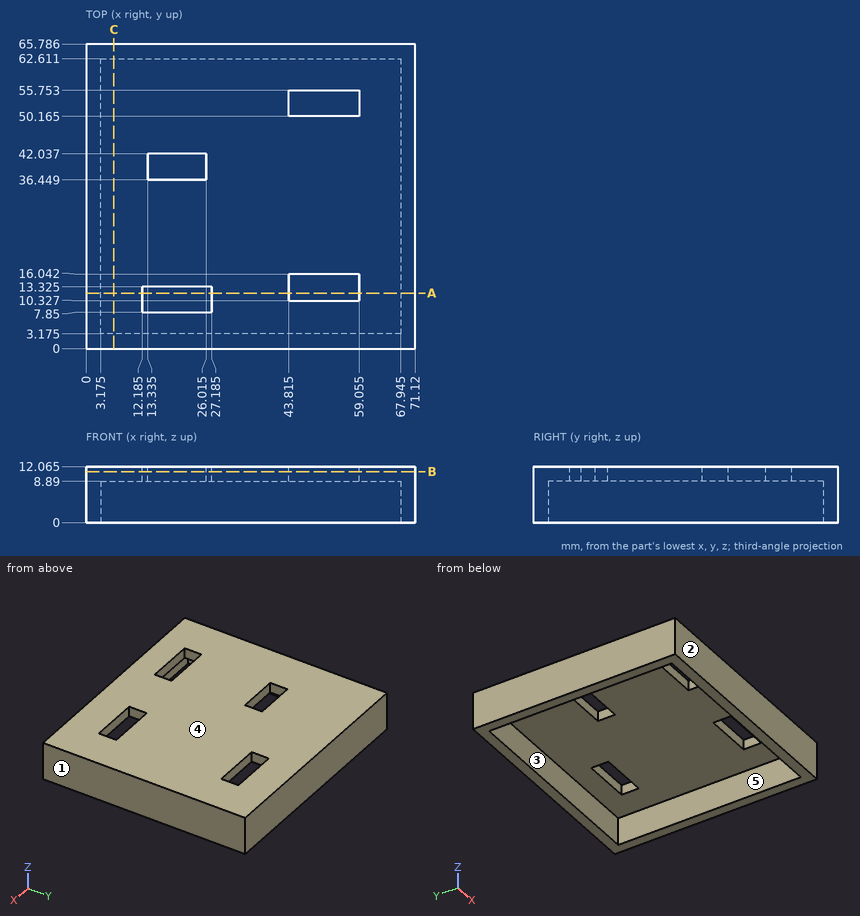
Study the drawing (mm; zero at the part's minimum x, y, z) and answer. A direction names the side the tool comes from. Give positions to 0.01 mm unless a question says otherwise; leave off trailing zeros. Write each loop counter-clockwise with the first axis right and the second up, starting at its lowest first coordinate (ties: lowest second). Pieces come first, ordered by that corner, then holes.
Item 1: Which of the six approach directions +Z, -Z, +X, -X, +Y, -Y give full straight-line access (tool end or side, diameter ignored) to the marked faces 4 and 5?
Item 2: Section B-B, the plane z = 11 is taken. Count the separate pieces of the cut face and the enclosed holes in it, plus the area to 3 significant figures.
Item 3: Flat-ended cylindrical pins translate along their axes: P1, Ø3.5, axis at y = 52, z = 11, coming from the -X side; P2, Ø8, axis at x = 35, y = 24.5, coming from the -Z side. Find the tip coordinate at first contact, or state that the pin passes through.
Item 4: Section A-A, the plane y = 12 is taken. Write down the section's boundary in (x, z) (3 decimals), plus the area to 3 significant figures.
Item 5: Determine the mould class of the marked faces 1, 2 and 3 for opening direction Y: released by +Y, released by -Y, zero draft, split by the parting line, or undercut.
Item 6: Find the intervals of material crossed by line 1 along X through (y, z) = (11.5, 10.75) (3 decimals); line 2 along Y through (x, z) = (32.5, 5.5) (3 decimals); line 3 along X through (y, z) = (8, 4) (3 decimals), in increasing order.
Item 7: Section C-C, the plane x = 6 is taken. Write down the section's boundary in (y, z) (3 decimals), plus the area to 3 significant figures.
Completed:
1. face 4: +Z, +X, -X, +Y, -Y
1. face 5: -Z
2. separate pieces: 1
2. enclosed holes: 4
2. area: 4,350 mm2
3. P1: stops at x = 0
3. P2: stops at z = 8.89
4. outline: (0, 0) - (3.175, 0) - (3.175, 8.89) - (12.185, 8.89) - (12.185, 12.065) - (0, 12.065) - close; (27.185, 8.89) - (43.815, 8.89) - (43.815, 12.065) - (27.185, 12.065) - close; (59.055, 8.89) - (67.945, 8.89) - (67.945, 0) - (71.12, 0) - (71.12, 12.065) - (59.055, 12.065) - close
4. area: 186 mm2
5. face 1: zero draft
5. face 2: released by -Y
5. face 3: undercut
6. line 1: x = 0 to 12.185, 27.185 to 43.815, 59.055 to 71.12
6. line 2: y = 0 to 3.175, 62.611 to 65.786
6. line 3: x = 0 to 3.175, 67.945 to 71.12
7. outline: (0, 0) - (3.175, 0) - (3.175, 8.89) - (62.611, 8.89) - (62.611, 0) - (65.786, 0) - (65.786, 12.065) - (0, 12.065) - close
7. area: 265 mm2
